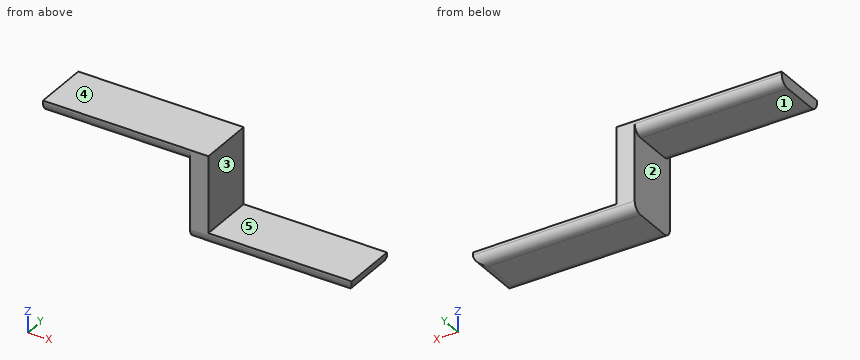
```python
from build123d import *

# Parameters (mm, degrees)
SKETCH2_W           = 12.7
SKETCH2_H           = 44.45
BOSS_EXTRUDE1_DEPTH = 38.1
FILLET1_R           = 6.35


with BuildPart() as part:
    # Sketch2 → Boss-Extrude1 (new body)
    with BuildSketch(Plane(origin=(0, 0, 0), x_dir=(1, 0, 0), z_dir=(0, 1, 0))):
        Polygon((0, 8.255), (0, 0), (114.3, 0), (114.3, 8.255), (101.6, 8.255), align=None)
        with Locations((107.95, 30.48)):
            Rectangle(SKETCH2_W, SKETCH2_H)
        Polygon((101.6, 52.705), (114.3, 52.705), (213.36, 52.705), (213.36, 60.96), (101.6, 60.96), align=None)
    extrude(amount=BOSS_EXTRUDE1_DEPTH)

    # Fillet1
    fillet1_edges = [part.edges().sort_by_distance(p)[0] for p in [
        (50.8, 0, -8.255),
        (157.48, 0, -60.96),
        (213.36, 19.05, -60.96),
        (157.48, 38.1, -60.96),
        (50.8, 38.1, -8.255),
    ]]
    fillet(fillet1_edges, radius=FILLET1_R)


solid = part.part
```
Could you check a few things on this model? Use its own coordinates, in mm. Face numbers are marked on the shaded views. A direction names the side the tool comes from. Round coordinates to 2 decimals unless told otherwise and drop trailing zeros. Order: outer loops, then holes, each group sorted by start corner. A loop starts at its lowest first (then second) coordinate and runs counter-clockwise, first axis right, second up. Notation, with made-up numbers: M -6,16 L 27,16 A19 ccw 27,40 Z; hole C -26,10.5 d1. An arc over 180 degrees is marked long. One line per question, with ' | ' between items. Start each with the question number.
(1) Suppose I cut it at A-A on y = 15. List the corners of the cut face in (x, z) for me (3 decimals), then the cut area to 3 significant figures.
(2) Thinking about a two-plate mould opening in X: for the marked faces 1, 2 and 3, which applies, +X half, -X half, draft (parallel to the pull), parting line (faces both ways), or undercut?
(3) Suppose I cut it at B-B on x = 179. List the corners of the cut face in (y, z) for me (3 decimals), then the cut area to 3 significant figures.
(4) For P1, Ø1, axis at y = 15.5, z = -20, coming from the +X side; P2, Ø11.5, axis at x = 161.5, y = 24.5, coming from the +Z side (3 decimals); P3, Ø19, axis at y = 28.5, z = -30, coming from the -X side, each with a flat end and sliding along its axis, tell me the tip position at first contact or that it passes through.
(5) For the marked faces 4 and 5, which set-ups out of +Z, -Z, +X, -X, +Y, -Y let a thin tool reach every point of the face, with its end or its side?
(6) Suppose I cut it at C-C on z = -50.5. List the corners of the cut face in (x, y) for me, then the cut area to 3 significant figures.
(7) Please list where these lines run through material, in increasing order: line 1 along Z through (x, y) = (54, 11) (3 decimals); line 2 along X through (y, z) = (36, -5); line 3 along X through (y, z) = (28.5, -36).
Geometry results:
1) outline: M 0,-8.255 L 101.6,-8.255 L 101.6,-60.96 L 207.01,-60.96 A6.35 ccw 213.36,-54.61 L 213.36,-52.705 L 114.3,-52.705 L 114.3,0 L 0,0 Z | area: 2,420 mm²
2) face 1: draft | face 2: -X half | face 3: +X half
3) outline: M 0,-54.61 A6.35 ccw 6.35,-60.96 L 31.75,-60.96 A6.35 ccw 38.1,-54.61 L 38.1,-52.705 L 0,-52.705 Z | area: 297 mm²
4) P1: x = 114.3 | P2: z = -52.705 | P3: x = 101.6
5) face 4: +Z, +X, -X, +Y, -Y | face 5: +Z, +X, +Y, -Y
6) outline: M 101.6,0 L 114.3,0 L 114.3,38.1 L 101.6,38.1 Z | area: 484 mm²
7) line 1: -8.255 to 0 | line 2: 0 to 114.3 | line 3: 101.6 to 114.3
